Here's the drawing with two shaded views (mm, measured from the low corner). I have some questions. Give positions to 0.01 mm unless a question says otherwise; leave off trailing zeros. Loops run counter-clockwise (first coordinate to the right, second up) from the corner with the lowest first, then second, coordinate; pieces in that order, holes last. Notation, with made-up numbers: M 40,1 L 78,1 A32 ccw 78,32 Z; hole C 68,-35 d5. An arc over 180 degrees is marked long. Write item = value, one per line. Start each with the question number.
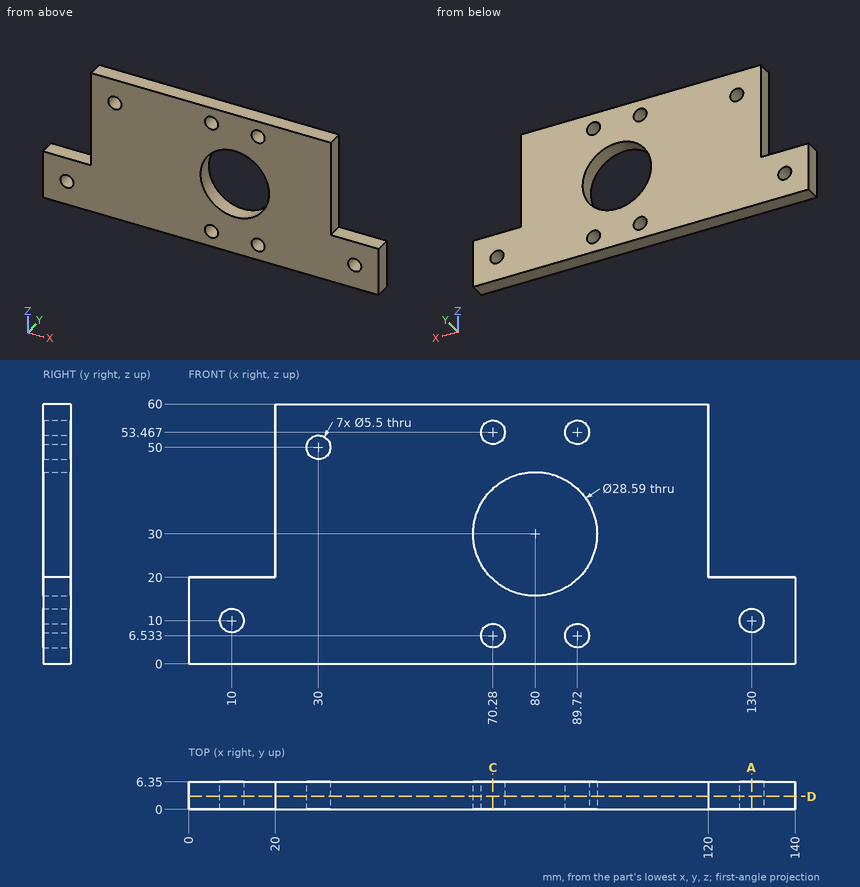
Q1. If we section it at A-A, the plane x = 130: List the corners of the cut face in (y, z) for me.
Q2. Will these pins go through, and if not, where does the flat tip stop? pin 1 (2 mm diameter, centred on y = 3, z = 32.5, fed in from -X); pin 2 (1.9 mm diameter, centred on y = 3, z = 40, fed in from +X); pin 3 (1.9 mm diameter, centred on x = 126, y = 4, fed in from +Z).
Q3. If we section it at D-D, the plane y = 3: State how many separate pieces and enclosed holes the cut face has, then the cut area to 3 significant figures.
Q4. If we section it at C-C, the plane x = 70.28: List the corners of the cut face in (y, z) for me, then the cut area to 3 significant figures.
Q5. If I drill on line 1 along X through (y, z) = (4, 10); line 2 along X through (y, z) = (0.75, 52) (1 decimal); line 3 along Z through (x, y) = (30, 3), over which ranges is the centre line in solid material (lowest first)?
Resolved:
q1.outline = M 0,0 L 6.35,0 L 6.35,7.25 L 0,7.25 Z; M 0,12.75 L 6.35,12.75 L 6.35,20 L 0,20 Z
q2.pin_1 = 20
q2.pin_2 = 120
q2.pin_3 = 20
q3.separate_pieces = 1
q3.enclosed_holes = 8
q3.area = 5,990 mm²
q4.outline = M 0,0 L 6.35,0 L 6.35,3.78 L 0,3.78 Z; M 0,9.28 L 6.35,9.28 L 6.35,19.52 L 0,19.52 Z; M 0,40.48 L 6.35,40.48 L 6.35,50.72 L 0,50.72 Z; M 0,56.22 L 6.35,56.22 L 6.35,60 L 0,60 Z
q4.area = 178 mm²
q5.line_1 = 0 to 7.25, 12.75 to 127.25, 132.75 to 140
q5.line_2 = 20 to 28.1, 31.9 to 68, 72.6 to 87.4, 92 to 120
q5.line_3 = 0 to 47.25, 52.75 to 60
